Geometry: final body of the model. Coordinates: model frame, mm. A direction names the side the tool comes from. Give positions to 0.01 mm unless a question says otherwise; leave off trailing zeros. Order: outer loops, then holes, each group sorted by start corner. A loop starts at its lowest first (then second) coordinate and runs counter-clockwise, first axis right, second up. Notation, with made-up numbers: (-12, 78) - (3, 78) arc R17 ccw to (3, 100) - close; hole circle Ø10 at (1.25, 66). An arc over 180 degrees is marked (long way). Write item = value, one per line. Start each with the question number.
from build123d import *

# Parameters (mm, degrees)
SKETCH_W        = 43
SKETCH_H        = 21
SKETCH_W_2      = 21
SKETCH_H_2      = 43
PAD_DEPTH       = 3
SKETCH001_W     = 4
SKETCH001_H     = 22
SKETCH001_W_2   = 22
SKETCH001_H_2   = 4
PAD001002_DEPTH = 24.5
SKETCH002_W     = 22
SKETCH002_H     = 29
SKETCH002_W_2   = 29
SKETCH002_H_2   = 22
PAD001003_DEPTH = 3
SKETCH003_R     = 1.5
POCKET_DEPTH    = 5


with BuildPart() as part:
    # Sketch → Pad (new body, symmetric)
    with BuildSketch(Plane.XY):
        Polygon((-14.5, 68), (14.5, 68), (14.5, 14.5), (68, 14.5), (68, -14.5), (14.5, -14.5), (14.5, -68), (-14.5, -68), (-14.5, -14.5), (-68, -14.5), (-68, 14.5), (-14.5, 14.5), align=None)
        with Locations((39, 0)):
            Rectangle(SKETCH_W, SKETCH_H, mode=Mode.SUBTRACT)
        with Locations((0, 39)):
            Rectangle(SKETCH_W_2, SKETCH_H_2, mode=Mode.SUBTRACT)
        with Locations((-39, 0)):
            Rectangle(SKETCH_W, SKETCH_H, mode=Mode.SUBTRACT)
        with Locations((0, -39)):
            Rectangle(SKETCH_W_2, SKETCH_H_2, mode=Mode.SUBTRACT)
    extrude(amount=PAD_DEPTH, both=True)

    # Sketch001 → Pad001002 (new body)
    with BuildSketch(Plane(origin=(0, 0, -3), x_dir=(1, 0, 0), z_dir=(0, 0, -1))):
        with Locations((12.5, 49.5)):
            Rectangle(SKETCH001_W, SKETCH001_H)
        with Locations((-12.5, 49.5)):
            Rectangle(SKETCH001_W, SKETCH001_H)
        with Locations((-12.5, -49.5)):
            Rectangle(SKETCH001_W, SKETCH001_H)
        with Locations((12.5, -49.5)):
            Rectangle(SKETCH001_W, SKETCH001_H)
        with Locations((-49.5, 12.5)):
            Rectangle(SKETCH001_W_2, SKETCH001_H_2)
        with Locations((-49.5, -12.5)):
            Rectangle(SKETCH001_W_2, SKETCH001_H_2)
        with Locations((49.5, -12.5)):
            Rectangle(SKETCH001_W_2, SKETCH001_H_2)
        with Locations((49.5, 12.5)):
            Rectangle(SKETCH001_W_2, SKETCH001_H_2)
    extrude(amount=PAD001002_DEPTH)

    # Sketch002 → Pad001003 (new body)
    with BuildSketch(Plane(origin=(0, 0, -27.5), x_dir=(1, 0, 0), z_dir=(0, 0, -1))):
        with Locations((-49.5, 0)):
            Rectangle(SKETCH002_W, SKETCH002_H)
        with Locations((0, 49.5)):
            Rectangle(SKETCH002_W_2, SKETCH002_H_2)
        with Locations((49.5, 0)):
            Rectangle(SKETCH002_W, SKETCH002_H)
        with Locations((0, -49.5)):
            Rectangle(SKETCH002_W_2, SKETCH002_H_2)
    extrude(amount=-PAD001003_DEPTH)

    # Sketch003 → Pocket (cut)
    with BuildSketch(Plane(origin=(0, 0, -27.5), x_dir=(1, 0, 0), z_dir=(0, 0, -1))):
        with Locations((0, -48.5)):
            Circle(SKETCH003_R)
        with Locations((-48.5, 0)):
            Circle(SKETCH003_R)
        with Locations((0, 48.5)):
            Circle(SKETCH003_R)
        with Locations((48.5, 0)):
            Circle(SKETCH003_R)
    extrude(amount=-POCKET_DEPTH, mode=Mode.SUBTRACT)


solid = part.part
Q1. Pull-direction query (Y, two-part tool) for faces 1 (the flat face through (0, 64, -3)), 2 (the flat face through (0, 68, 0)), 3 (the flat face through (0, -60.5, 0)); classes: +Y half, -Y half, draft (parallel to the pull), parting line (faces both ways), or undercut.
Q2. Contact query for flat-ended pins moving along their axis: pin 1 (9 mm diameter, centred on x = 39, z = -8.5, fed in from +Y); pin 2 (4 mm diameter, centred on x = -65, y = -4, fed in from -Z); pin 3 (10.5 mm diameter, centred on x = -46, y = 1.5, fed in from +Z). Output: stop coordinate, or through.
Q3. Material intervals for line 1 along Y through (x, z) = (0, -25.5); line 2 along Y through (x, z) = (21, -2), sorted ascending. Write a range as from..to.
Q4. Set-up query: faces 4 (the flat face through (0, 17.5, 0)), 5 (the flat face through (-48, 14.5, -9)), 6 (the flat face through (0, 38.5, -25)). Return all of +Z, -Z, +X, -X, +Y, -Y with unobstructed straight access to the full face (end or side cutting, diameter ignored); none if empty.
Q5. Section C-C, the plane z = -14. Count the separate pieces of the cut face and the enclosed holes in it, then the cut area to 3 significant figures.
Q6. Section A-A, the plane y = 8.5. Return the cut outline in (x, z), then the cut area to 3 significant figures.
Q7. Section B-B, the plane x = -20. Return the cut outline in (y, z).
The answers:
q1.face_1 = draft
q1.face_2 = +Y half
q1.face_3 = undercut
q2.pin_1 = 14.5
q2.pin_2 = -3
q2.pin_3 = -24.5
q3.line_1 = -60.5..-50, -47..-38.5, 38.5..47, 50..60.5
q3.line_2 = -14.5..-10.5, 10.5..14.5
q4.face_4 = +Z, -Z
q4.face_5 = +Z, -Z, -X, +Y
q4.face_6 = -Z, +X, -X
q5.separate_pieces = 8
q5.enclosed_holes = 0
q5.area = 704 mm²
q6.outline = (-68, -3) - (-60.5, -3) - (-60.5, 3) - (-68, 3) - close; (-60.5, -27.5) - (-38.5, -27.5) - (-38.5, -24.5) - (-60.5, -24.5) - close; (-17.5, -3) - (17.5, -3) - (17.5, 3) - (-17.5, 3) - close; (38.5, -27.5) - (60.5, -27.5) - (60.5, -24.5) - (38.5, -24.5) - close; (60.5, -3) - (68, -3) - (68, 3) - (60.5, 3) - close
q6.area = 432 mm²
q7.outline = (-14.5, -3) - (-10.5, -3) - (-10.5, 3) - (-14.5, 3) - close; (10.5, -3) - (14.5, -3) - (14.5, 3) - (10.5, 3) - close
